from build123d import *

# Parameters (mm, degrees)
BOSS_EXTRUDE1_DEPTH     = 10
SKETCH2_W               = 17.2
SKETCH2_H               = 43
CUT_EXTRUDE1_DEPTH      = 72.414284285
SKETCH3_W               = 90
SKETCH3_H               = 34
SKETCH3_W_2             = 80
SKETCH3_H_2             = 24
BOSS_EXTRUDE3_DEPTH     = 15
SKETCH4_W               = 49.6
SKETCH4_H               = 5
BOSS_EXTRUDE4_DEPTH     = 10
SKETCH5_W               = 15
SKETCH5_H               = 22
BOSS_EXTRUDE5_DEPTH     = 5
SKETCH6_W               = 90
SKETCH6_H               = 77
BOSS_EXTRUDE6_DEPTH     = 15
BOSS_EXTRUDE8_DEPTH     = 39
CHAMFER1_SIZE           = 64
CHAMFER1_SIZE_2         = 3.354097874
CHAMFER2_SIZE           = 64
CHAMFER2_SIZE_2         = 11.405813635
CHAMFER3_SIZE           = 64
CHAMFER3_SIZE_2         = 13.775745352
CUT_EXTRUDE3_DEPTH      = 95.500525601
CUT_EXTRUDE3_DEPTH_BACK = 95.500525601
SKETCH10_W              = 50
SKETCH10_H              = 27
SKETCH11_W              = 45.5
SKETCH11_H              = 10.5
CUT_EXTRUDE4_DEPTH      = 7.5
SKETCH14_W              = 2.05
SKETCH14_H              = 10.5
BOSS_EXTRUDE9_DEPTH     = 15
SKETCH15_R              = 8
CUT_EXTRUDE5_DEPTH      = 122.227059686
CUT_EXTRUDE6_DEPTH      = 2.5
CUT_EXTRUDE7_REACH      = 97.373
SKETCH18_W              = 29.6
SKETCH18_H              = 45
CUT_EXTRUDE8_DEPTH      = 15
SKETCH21_W              = 29.6
SKETCH21_H              = 35
BOSS_EXTRUDE10_DEPTH    = 2.5
SKETCH22_W              = 90
SKETCH22_H              = 72
CUT_EXTRUDE9_DEPTH      = 54


with BuildPart() as part:
    # Sketch1 → Boss-Extrude1 (new body)
    with BuildSketch(Plane(origin=(0, 0, 0), x_dir=(1, 0, 0), z_dir=(0, 1, 0))):
        with BuildLine():
            Line((-35, 50), (35, 50))
            ThreePointArc((35, 50), (45.606601718, 45.606601718), (50, 35))
            Line((50, 35), (50, -35))
            ThreePointArc((50, -35), (45.606601718, -45.606601718), (35, -50))
            Line((35, -50), (-35, -50))
            ThreePointArc((-35, -50), (-45.606601718, -45.606601718), (-50, -35))
            Line((-50, -35), (-50, 35))
            ThreePointArc((-50, 35), (-45.606601718, 45.606601718), (-35, 50))
        make_face()
    extrude(amount=BOSS_EXTRUDE1_DEPTH)

    # Sketch2 → Cut-Extrude1 (cut, through all)
    with BuildSketch(Plane(origin=(0, 10, 0), x_dir=(1, 0, 0), z_dir=(0, 1, 0))):
        with Locations((-33.4, 18.5)):
            Rectangle(SKETCH2_W, SKETCH2_H)
        with Locations((33.4, 18.5)):
            Rectangle(SKETCH2_W, SKETCH2_H)
    extrude(amount=-CUT_EXTRUDE1_DEPTH, mode=Mode.SUBTRACT)

    # Sketch3 → Boss-Extrude3 (add)
    with BuildSketch(Plane(origin=(0, 10, 0), x_dir=(1, 0, 0), z_dir=(0, 1, 0))):
        with Locations((0, -20)):
            Rectangle(SKETCH3_W, SKETCH3_H)
        with Locations((0, -20)):
            Rectangle(SKETCH3_W_2, SKETCH3_H_2, mode=Mode.SUBTRACT)
    extrude(amount=BOSS_EXTRUDE3_DEPTH)

    # Sketch4 → Boss-Extrude4 (add)
    with BuildSketch(Plane(origin=(0, 10, 0), x_dir=(1, 0, 0), z_dir=(0, 1, 0))):
        with Locations((0, 10)):
            Rectangle(SKETCH4_W, SKETCH4_H)
        with Locations((0, 27)):
            Rectangle(SKETCH4_W, SKETCH4_H)
    extrude(amount=BOSS_EXTRUDE4_DEPTH)

    # Sketch5 → Boss-Extrude5 (add)
    with BuildSketch(Plane(origin=(0, 20, 0), x_dir=(1, 0, 0), z_dir=(0, 1, 0))):
        with Locations((-17.3, 18.5)):
            Rectangle(SKETCH5_W, SKETCH5_H)
        with Locations((17.3, 18.5)):
            Rectangle(SKETCH5_W, SKETCH5_H)
    extrude(amount=BOSS_EXTRUDE5_DEPTH)

    # Sketch6 → Boss-Extrude6 (add)
    with BuildSketch(Plane(origin=(0, 10, 0), x_dir=(1, 0, 0), z_dir=(0, 1, 0))):
        with BuildLine():
            Line((-50, 35), (-50, -35))
            ThreePointArc((-50, -35), (-45.606601718, -45.606601718), (-35, -50))
            Line((-35, -50), (35, -50))
            ThreePointArc((35, -50), (45.606601718, -45.606601718), (50, -35))
            Line((50, -35), (50, 35))
            ThreePointArc((50, 35), (45.606601718, 45.606601718), (35, 50))
            Line((35, 50), (-35, 50))
            ThreePointArc((-35, 50), (-45.606601718, 45.606601718), (-50, 35))
        make_face()
        with Locations((0, 1.5)):
            Rectangle(SKETCH6_W, SKETCH6_H, mode=Mode.SUBTRACT)
    extrude(amount=BOSS_EXTRUDE6_DEPTH)

    # Sketch9 → Boss-Extrude8 (add)
    with BuildSketch(Plane(origin=(0, 25, 0), x_dir=(1, 0, 0), z_dir=(0, 1, 0))):
        with BuildLine():
            Line((-50, 35), (-50, -35))
            ThreePointArc((-50, -35), (-45.606601718, -45.606601718), (-35, -50))
            Line((-35, -50), (35, -50))
            ThreePointArc((35, -50), (45.606601718, -45.606601718), (50, -35))
            Line((50, -35), (50, 35))
            ThreePointArc((50, 35), (45.606601718, 45.606601718), (35, 50))
            Line((35, 50), (-35, 50))
            ThreePointArc((-35, 50), (-45.606601718, 45.606601718), (-50, 35))
        make_face()
        with BuildLine():
            Line((-45, 35), (-45, -32))
            Line((-45, -32), (45, -32))
            Line((45, -32), (45, 35))
            ThreePointArc((45, 35), (44.659258263, 37.588190451), (43.660254038, 40))
            Line((43.660254038, 40), (-43.660254038, 40))
            ThreePointArc((-43.660254038, 40), (-44.659258263, 37.588190451), (-45, 35))
        make_face(mode=Mode.SUBTRACT)
    extrude(amount=BOSS_EXTRUDE8_DEPTH)

    # Chamfer1
    # the kernel refuses this chamfer: 64, 3.354097874 mm, written as the material it takes off along each edge
    with BuildSketch(Plane(origin=(-35, 64, 50), x_dir=(0, -0.9999979738662979, 0.002013023422382214), z_dir=(1, 0, 0)), Plane(origin=(50, 64, 35), x_dir=(0.002013023422382214, -0.9999979738662979, 0), z_dir=(0, 0, -1)), Plane(origin=(-50, 64, -35), x_dir=(-0.002013023422382214, -0.9999979738662979, 0), z_dir=(0, 0, 1)), Plane(origin=(35, 64, -50), x_dir=(0, -0.9999979738662979, -0.002013023422382214), z_dir=(-1, 0, 0))) as chamfer1_piece_1:
        Polygon((CHAMFER1_SIZE * 0.999997973866, CHAMFER1_SIZE * 0.00201302342238), (-CHAMFER1_SIZE_2 * 0.00201302342245, CHAMFER1_SIZE_2 * 0.9999979739), (0, 0), align=None)
    extrude(amount=70, mode=Mode.SUBTRACT)
    with BuildSketch(Plane(origin=(35, 64, 35), x_dir=(0, 0, 1), z_dir=(-1, 0, 0))) as chamfer1_piece_2:
        Polygon((15, -CHAMFER1_SIZE), (15 - CHAMFER1_SIZE_2, 0), (15, 0), align=None)
    revolve(axis=Axis((35, 64, 35), (0, 1, 0)), revolution_arc=90, mode=Mode.SUBTRACT)
    with BuildSketch(Plane(origin=(-35, 64, 35), x_dir=(-1, 0, 0), z_dir=(0, 0, -1))) as chamfer1_piece_3:
        Polygon((15, -CHAMFER1_SIZE), (15 - CHAMFER1_SIZE_2, 0), (15, 0), align=None)
    revolve(axis=Axis((-35, 64, 35), (0, 1, 0)), revolution_arc=90, mode=Mode.SUBTRACT)
    with BuildSketch(Plane(origin=(35, 64, -35), x_dir=(1, 0, 0), z_dir=(0, 0, 1))) as chamfer1_piece_4:
        Polygon((15, -CHAMFER1_SIZE), (15 - CHAMFER1_SIZE_2, 0), (15, 0), align=None)
    revolve(axis=Axis((35, 64, -35), (0, 1, 0)), revolution_arc=90, mode=Mode.SUBTRACT)
    with BuildSketch(Plane(origin=(-35, 64, -35), x_dir=(0, 0, -1), z_dir=(1, 0, 0))) as chamfer1_piece_5:
        Polygon((15 - CHAMFER1_SIZE_2, 0), (15, -CHAMFER1_SIZE), (15, 0), align=None)
    revolve(axis=Axis((-35, 64, -35), (0, 1, 0)), revolution_arc=90, mode=Mode.SUBTRACT)

    # Chamfer2
    # the kernel refuses this chamfer: 64, 11.405813635 mm, written as the material it takes off along each edge
    with BuildSketch(Plane(origin=(201.306482971, 64, -46.645902126), x_dir=(0, -0.9982575003065525, -0.05900816114499234), z_dir=(-1, 0, 0))) as chamfer2_piece_1:
        Polygon((CHAMFER2_SIZE * 0.999977671636, CHAMFER2_SIZE * 0.0066825316561), (-CHAMFER2_SIZE_2 * 0.0590081611462, CHAMFER2_SIZE_2 * 0.998257500326), (0, 0), align=None)
    extrude(amount=402.612965942, mode=Mode.SUBTRACT)

    # Chamfer3
    # the kernel refuses this chamfer: 64, 13.775745352 mm, written as the material it takes off along each edge
    with BuildSketch(Plane(origin=(-201.265469314, 64, 46.645902126), x_dir=(0, -0.9981787050157903, 0.06032638604292662), z_dir=(1, 0, 0))) as chamfer3_piece_1:
        Polygon((CHAMFER3_SIZE * 0.999967974892, CHAMFER3_SIZE * 0.00800307379952), (-CHAMFER3_SIZE_2 * 0.060326386045, CHAMFER3_SIZE_2 * 0.99817870505), (0, 0), align=None)
    extrude(amount=402.530938629, mode=Mode.SUBTRACT)

    # Sketch10 → Cut-Extrude3 (cut, two sides: drawn at the far end of the back side and taken through both)
    with BuildSketch(Plane(origin=(0, 1.307501734, 0), x_dir=(0, 0, 1), z_dir=(-1, 0, 0)).offset(-CUT_EXTRUDE3_DEPTH_BACK)):
        with Locations((-22.129843227, 49.192498266)):
            Rectangle(SKETCH10_W, SKETCH10_H)
    extrude(amount=CUT_EXTRUDE3_DEPTH + CUT_EXTRUDE3_DEPTH_BACK, mode=Mode.SUBTRACT)

    # Sketch11 → Cut-Extrude4 (cut)
    with BuildSketch(Plane(origin=(0, 10, 0), x_dir=(1, 0, 0), z_dir=(0, 1, 0))):
        with Locations((0, 34.75)):
            Rectangle(SKETCH11_W, SKETCH11_H)
    extrude(amount=-CUT_EXTRUDE4_DEPTH, mode=Mode.SUBTRACT)

    # Sketch14 → Boss-Extrude9 (add)
    with BuildSketch(Plane(origin=(0, 10, 0), x_dir=(1, 0, 0), z_dir=(0, 1, 0))):
        with Locations((-23.775, 34.75)):
            Rectangle(SKETCH14_W, SKETCH14_H)
        with Locations((23.775, 34.75)):
            Rectangle(SKETCH14_W, SKETCH14_H)
    extrude(amount=BOSS_EXTRUDE9_DEPTH)

    # Sketch15 → Cut-Extrude5 (cut, through all)
    with BuildSketch(Plane.XY.offset(-40)):
        with Locations((-12.75, 12.75)):
            Circle(SKETCH15_R)
        with Locations((12.75, 12.75)):
            Circle(SKETCH15_R)
    extrude(amount=-CUT_EXTRUDE5_DEPTH, mode=Mode.SUBTRACT)

    # Sketch17 → Cut-Extrude6 (cut)
    with BuildSketch(Plane(origin=(0, 0, -29.5), x_dir=(-1, 0, 0), z_dir=(0, 0, -1))):
        Polygon((-9.8, 25), (-22.75, 25), (-22.75, 2.5), (22.75, 2.5), (22.75, 25), (9.8, 25), (9.8, 20), (-9.8, 20), align=None)
    extrude(amount=-CUT_EXTRUDE6_DEPTH, mode=Mode.SUBTRACT)

    # Cut-Extrude7: up to this face of the body (flat: up to its plane)
    cut_extrude7_end = Plane(part.part.faces().sort_by_distance((0, 10, -18.5))[0])
    # Sketch18 → Cut-Extrude7 (cut, up to the picked face)
    with BuildSketch(Plane.XZ, mode=Mode.PRIVATE) as cut_extrude7_sk1:
        with Locations((0, -4.5)):
            Rectangle(SKETCH18_W, SKETCH18_H)
    cut_extrude7_tool1 = split(extrude(cut_extrude7_sk1.sketch, amount=-CUT_EXTRUDE7_REACH, mode=Mode.PRIVATE), bisect_by=cut_extrude7_end, keep=Keep.BOTH, mode=Mode.PRIVATE)
    add(cut_extrude7_tool1.solids().sort_by(Axis((0, 0, -4.5), (0, 1, 0)))[0], mode=Mode.SUBTRACT)

    # Sketch20 → Cut-Extrude8 (cut)
    with BuildSketch(Plane.XZ.offset(-25)):
        with BuildLine():
            Line((-45, -35), (-45, -40))
            Line((-45, -40), (-43.660254038, -40))
            ThreePointArc((-43.660254038, -40), (-44.659258263, -37.588190451), (-45, -35))
        make_face()
        with BuildLine():
            Line((45, -40), (45, -35))
            ThreePointArc((45, -35), (44.659258263, -37.588190451), (43.660254038, -40))
            Line((43.660254038, -40), (45, -40))
        make_face()
    extrude(amount=-CUT_EXTRUDE8_DEPTH, mode=Mode.SUBTRACT)

    # Sketch21 → Boss-Extrude10 (add)
    with BuildSketch(Plane.XZ):
        with Locations((0, 0.5)):
            Rectangle(SKETCH21_W, SKETCH21_H)
    extrude(amount=-BOSS_EXTRUDE10_DEPTH)

    # Sketch22 → Cut-Extrude9 (cut)
    with BuildSketch(Plane(origin=(0, 64, 0), x_dir=(1, 0, 0), z_dir=(0, 1, 0))):
        with Locations((0, 4)):
            Rectangle(SKETCH22_W, SKETCH22_H)
    extrude(amount=-CUT_EXTRUDE9_DEPTH, mode=Mode.SUBTRACT)


solid = part.part
Work out the finished part from the listing and answer in its coordinate system (mm). A direction names the side the tool comes from. Give positions to 0.01 mm unless a question says otherwise; leave off trailing zeros. Order: outer loops, then holes, each group sorted by start corner. A loop starts at its lowest first (then second) coordinate and runs counter-clockwise, first axis right, second up. Notation, with made-up numbers: (44, 16) -> (53, 16) arc R15 ccw to (53, 32) -> close; hole circle Ø9 at (68, 60). An arc over 180 degrees is marked (long way). Answer as a JSON object with one key per item and string values. Group by question number.
1. Section A-A on z = -11 is taken. Determine the outline of the cut face in (x, y).
2. Section D-D on y = 8 is taken. Count the separate pieces of the cut face and the enclosed holes in it, plus the area to 3 significant figures.
3. Section C-C on x = -28.5 is taken. Determine the outline of the cut face in (y, z), plus the area to 3 significant figures.
4. Section B-B on y = 17 is taken. Determine the outline of the cut face in (x, z).
5. A tool of negligible diameter and unlimited length cuts with its end or side. For faces 1 (the flat face through (0, 37, -41)), 2 (the conical face through (47.77, 15.96, 41.13)), 3 (the flat face through (0, 1, -17)), 4 (the flat face through (14.8, 6, -5)), from which of +Z, -Z, +X, -X, +Y, -Y can it reach the whole face along a straight path? Write none if from no direction.
6. Flat-ended cylindrical pins translate along their axes: pin 1 Ø3 at (y, z) = (5, -1.5) entering from +X; pin 2 Ø16 at (x, y) = (5.5, 26.5) entering from -Z; pin 3 Ø10 at (y, z) = (17, 15.5) entering from -X. Find the tip coordinate at first contact, or state that the pin passes through.
7. The mould has two halves that part along Y. Classify faces 5 (the conical face through (47.964, 14.648, -40.873)), 6 (the flat face through (-19, 6, -27)), 7 (the cylindrical face through (-14.48, 4.94, -43.41)): released by +Y, released by -Y, zero draft, split by the parting line, or undercut.
8. Consider line 1 along X through (y, z) = (12.75, -42.25); line 2 along X through (y, z) = (12, -42); line 3 along Y through (x, z) = (12.75, -46). Determine where each line is inside the solid, lowest interval first. Write a range as [from, to].
Result sheet:
{
 "1": {"outline": "(-50, 0) -> (-42, 0) -> (-42, 10) -> (-45, 10) -> (-45, 37) -> (-48.06, 37) -> close; (-24.8, 0) -> (24.8, 0) -> (24.8, 10) -> (14.8, 10) -> (14.8, 2.5) -> (-14.8, 2.5) -> (-14.8, 10) -> (-24.8, 10) -> close; (42, 0) -> (50, 0) -> (48.06, 37) -> (45, 37) -> (45, 10) -> (42, 10) -> close"},
 "2": {"separate pieces": "2", "enclosed holes": "2", "area": "5,790 mm^2"},
 "3": {"outline": "(0, -50) -> (0.09, -50) -> (37, -41.47) -> (37, -40) -> (0, -40) -> close; (0, 3) -> (10, 3) -> (10, 32) -> (64, 32) -> (64, 32.87) -> (0.09, 50) -> (0, 50) -> close", "area": "1,110 mm^2"},
 "4": {"outline": "(-49.11, -35) arc R14.11 ccw to (-43.72, -46.09) -> (-19.53, -46.09) -> (-19.53, -40) -> (-45, -40) -> (-45, 32) -> (45, 32) -> (45, -40) -> (19.53, -40) -> (19.53, -46.09) -> (43.72, -46.09) arc R14.11 ccw to (49.11, -35) -> (49.11, 35) arc R14.11 ccw to (44.46, 45.46) -> (-44.46, 45.46) arc R14.11 ccw to (-49.11, 35) -> close; (-5.97, -46.09) -> (5.97, -46.09) -> (5.97, -40) -> (-5.97, -40) -> close"},
 "5": {"face 1": "-Z, +X, -X, +Y", "face 2": "+Z, +X, +Y", "face 3": "+Y, -Y", "face 4": "+Y"},
 "6": {"pin 1": "stops at x = 49.82", "pin 2": "stops at z = -45.74", "pin 3": "stops at x = -49.37"},
 "7": {"face 5": "released by +Y", "face 6": "zero draft", "face 7": "undercut"},
 "8": {"line 1": "x = [-47.36, -20.75], [-4.75, 4.75], [20.75, 47.36]", "line 2": "x = [-47.55, -20.71], [-4.79, 4.79], [20.71, 47.55]", "line 3": "y = [0, 4.75]"}
}
